```python
from build123d import *

# Parameters (mm, degrees)
BOSS_EXTRUDE1_DEPTH = 6


with BuildPart() as part:
    # Sketch1 → Boss-Extrude1 (new body)
    with BuildSketch(Plane.XY):
        with BuildLine():
            ThreePointArc((7.493997598, 22.8), (0, 28), (-7.493997598, 22.8))
            Line((-7.493997598, 22.8), (-14.051245496, 5.25))
            ThreePointArc((-14.051245496, 5.25), (0, -15), (14.051245496, 5.25))
            Line((14.051245496, 5.25), (7.493997598, 22.8))
        make_face()
        with BuildLine():
            Line((-4, 9.16515139), (-4, 5))
            Line((-4, 5), (4, 5))
            Line((4, 5), (4, 9.16515139))
            ThreePointArc((4, 9.16515139), (0, -10), (-4, 9.16515139))
        make_face(mode=Mode.SUBTRACT)
    extrude(amount=BOSS_EXTRUDE1_DEPTH)


solid = part.part
```
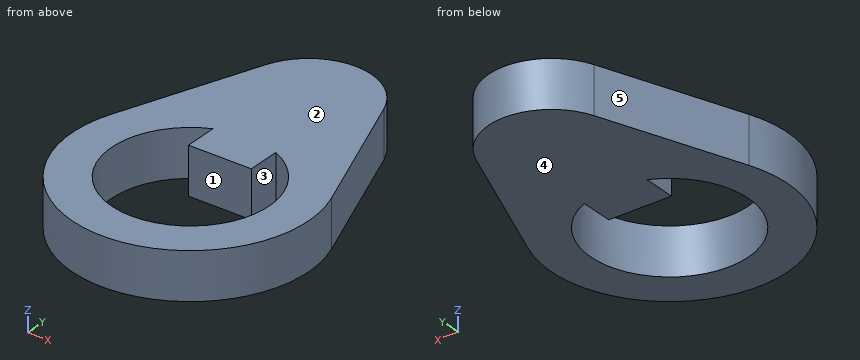
Here's how the part is built. I have some questions about the finished solid (model axes, mm). Face numbers are marked on the shaded views. A direction names the side the tool comes from. Coordinates: 2 decimals unless noted, no trailing zeros. Loops run counter-clockwise (first coordinate to the right, second up) from the corner with the lowest first, then second, coordinate; pieces in that order, holes last. Notation, with made-up numbers: (-3, 89.25) - (18, 89.25) arc R31 ccw to (18, 126.25) - close; hole circle Ø8 at (6.25, 45.25). An arc over 180 degrees is marked (long way). Answer as CSV lines item,"result".
Q1. For the marked faces 1 and 2, which set-ups out of +Z, -Z, +X, -X, +Y, -Y let a thin tool reach every point of the face, with its end or its side?
Response:
face 1,"+Z, -Z"
face 2,"+Z, +X, -X, +Y, -Y"
Q2. If we section it at A-A, the plane x = 0: Write out the boundary of the cut face in (y, z).
Response:
outline,"(-15, 0) - (-10, 0) - (-10, 6) - (-15, 6) - close; (5, 0) - (28, 0) - (28, 6) - (5, 6) - close"
Q3. If we section it at B-B, the plane y = 0: Write out the boundary of the cut face in (x, z).
Response:
outline,"(-15, 0) - (-10, 0) - (-10, 6) - (-15, 6) - close; (10, 0) - (15, 0) - (15, 6) - (10, 6) - close"
Q4. If we section it at C-C, the plane z = 0.7: Write out the boundary of the cut face in (x, y), and give its area (3 significant figures).
Response:
outline,"(-14.05, 5.25) arc R15 ccw (long way) to (14.05, 5.25) - (7.49, 22.8) arc R8 ccw to (-7.49, 22.8) - close; hole (-4, 5) - (-4, 9.17) arc R10 ccw (long way) to (4, 9.17) - (4, 5) - close"
area,"666 mm2"
Q5. For pin 1 (1 mm diameter, centred on x = -2.5, z = 2.5, fed in from -Y); pin 2 (1.5 mm diameter, centred on y = -2, z = 1, fed in from +X); pin 3 (2 mm diameter, centred on y = 7, z = 1.5, fed in from +X), each with a flat end and sliding along its axis, tell me the tip position at first contact or that it passes through.
Response:
pin 1,"y = -14.87"
pin 2,"x = 14.95"
pin 3,"x = 13.77"
Q6. If I drill on L1, parallel to Y at x = 0, z = 4.05; L2, parallel to X at y = 0, z = 3.5; L3, parallel to Y at x = -3.25, z = 5.7, over which ranges is the centre line in solid material (lowest first)? Write a range as [from, to].
Response:
L1,"[-15, -10], [5, 28]"
L2,"[-15, -10], [10, 15]"
L3,"[-14.64, -9.46], [5, 27.31]"
Q7. If we section it at D-D, the plane y = 15.5: Write out the boundary of the cut face in (x, z), and give its area (3 significant figures).
Response:
outline,"(-10.22, 0) - (10.22, 0) - (10.22, 6) - (-10.22, 6) - close"
area,"123 mm2"
Q8. We'd pull the mould along Y, two halves only. Please class the marked faces 3, 4 and 5: pulls with the +Y half, pulls with the -Y half, needs draft (parallel to the pull), parting line crosses it, or undercut.
Response:
face 3,"undercut"
face 4,"needs draft"
face 5,"pulls with the +Y half"
